Design review of the part built by this model. Coordinates are the model's own, in mm. A direction names the side the tool comes from. Coordinates: 2 decimals unless noted, no trailing zeros. Loops run counter-clockwise (first coordinate to the right, second up) from the corner with the lowest first, then second, coordinate; pieces in that order, holes last. Notation, with made-up numbers: (86, 21.25) - (131, 21.25) arc R27 ccw to (131, 54.25) - close; hole circle Ø8 at (4, -38). An arc over 180 degrees is marked (long way). Answer in a Markdown table with one row per item. Add a question column.
(1) We need section A-A, the plane z = 5. Write out the cut boundary in (x, y), plus the area to 3 significant figures.
(2) Clearance check with flat-ended pins moving along their axes: pin 1 (1.5 mm diameter, centred on x = 2.5, z = -10.5, fed in from -Y); pin 2 (1.2 mm diameter, centred on x = 0, y = 0, fed in from +Z); pin 3 (3 mm diameter, centred on x = -1, z = -13, fed in from +Y). State where each tip first meets the part, or that it passes through.
(3) We need section C-C, the plane z = -10.5. Write out the cut boundary in (x, y), plus the area to 3 significant figures.
(4) The part is to be moulded in two halves that separate along X. For faces 1 (the face through (2.155, -1.268, 0.14)), 2 (the face through (0.27, -1.22, 0.75)), 3 (the face through (0, -2.5, 0)), say which applies: released by +X, released by -X, zero draft, split by the parting line, or undercut.
(5) For faces 4 (the face through (-2.175, -1.233, 0.14)), 5 (the face through (1.45, 0.06, -12.96)), 6 (the face through (0, 0, -8)), list the 3-axis set-ups (+Z, -Z, +X, -X, +Y, -Y) from which the entire face can be reached by the end or side of a thin tool; tool diameter is ignored.
(6) To check wall thickness, follow L1, parallel to Y at x = 0, z = 5; L2, parallel to Z at x = -1.95, y = 0.75; L3, parallel to Z at x = 2.6, y = 0.2. State the ranges of each line that lie inside material, in increasing order. Write a range as [from, to].
from build123d import *

# Parameters (mm, degrees)
HEX_2_DEPTH                 = 10
TAP_DRILL_FOR_M3X0_5_TAP1_D = 2.5
SKETCH8_R                   = 1.45
THREAD_DEPTH                = 6
THREAD_DEPTH_BACK           = 2
INNERCHAMFER_SIZE           = 0.25


with BuildPart() as part:
    # Sketch1 → HEX 2 (new body, symmetric)
    with BuildSketch(Plane.XY):
        Polygon((2.886751346, 0), (1.443375673, 2.5), (-1.443375673, 2.5), (-2.886751346, 0), (-1.443375673, -2.5), (1.443375673, -2.5), align=None)
    extrude(amount=HEX_2_DEPTH, both=True)

    # Tap Drill for M3x0.5 Tap1 (through all)
    with Locations(Plane.XY.offset(10)):
        with Locations((0, 0)):
            Hole(TAP_DRILL_FOR_M3X0_5_TAP1_D / 2)

    # Sketch7 → HexChamfer (revolve, cut)
    with BuildSketch(Plane(origin=(0, 0, 0), x_dir=(1, 0, 0), z_dir=(0, 1, 0))):
        Polygon((-2.886751346, 10), (-2.886751346, 9.6), (-2.486751346, 10), align=None)
    hexchamfer = revolve(axis=Axis((0, 0, 15.266742202), (0, 0, -1)), mode=Mode.SUBTRACT)

    # Mirror1: HexChamfer across plane
    add(hexchamfer.mirror(Plane.XY), mode=Mode.SUBTRACT)

    # Sketch8 → Thread (add, two sides)
    with BuildSketch(Plane(origin=(0, 0, -10), x_dir=(-1, 0, 0), z_dir=(0, 0, -1))) as thread_sk:
        Circle(SKETCH8_R)
    extrude(amount=THREAD_DEPTH)
    extrude(thread_sk.sketch, amount=-THREAD_DEPTH_BACK)

    # InnerChamfer
    innerchamfer_edges = [part.edges().sort_by_distance(p)[0] for p in [
        (1.25, 0, 10),
        (1.45, 0, -10),
        (1.45, 0, -16),
    ]]
    chamfer(innerchamfer_edges, length=INNERCHAMFER_SIZE)


solid = part.part
Responses:
| question | item | result |
|---|---|---|
| 1 | outline | (-2.89, 0) - (-1.44, -2.5) - (1.44, -2.5) - (2.89, 0) - (1.44, 2.5) - (-1.44, 2.5) - close; hole circle Ø2.5 at (0, 0) |
| 1 | area | 16.7 mm2 |
| 2 | pin 1 | stops at y = -1.57 |
| 2 | pin 2 | stops at z = -8 |
| 2 | pin 3 | stops at y = 1.45 |
| 3 | outline | circle Ø2.9 at (0, 0) |
| 3 | area | 6.61 mm2 |
| 4 | face 1 | released by +X |
| 4 | face 2 | undercut |
| 4 | face 3 | zero draft |
| 5 | face 4 | +Z, -Z, -X, -Y |
| 5 | face 5 | -Z |
| 5 | face 6 | +Z |
| 6 | L1 | y = [-2.5, -1.25], [1.25, 2.5] |
| 6 | L2 | z = [-10, 10] |
| 6 | L3 | z = [-9.88, 9.88] |
